Work out the finished part from the listing and answer in its coordinate system (mm). A direction names the side the tool comes from. Round coordinates to 2 decimals unless told otherwise and drop trailing zeros. Order: outer loops, then holes, each group sorted by start corner. A loop starts at its lowest first (then second) coordinate and runs counter-clockwise, first axis right, second up. Notation, with made-up numbers: (-14, 1) - (35, 1) arc R28 cw to (35, 25) - close; hole circle Ø9 at (-8.5, 27). An arc over 180 degrees is marked (long way). Answer in a Markdown table with one row per item.
from build123d import *

# Parameters (mm, degrees)
F1_W     = 279.4
F1_H     = 482.6
F1_W_2   = 221.90693
F1_H_2   = 17.004371
F1_H_3   = 15.303909
F1_H_4   = 15.30391
F2_DEPTH = 25.4


with BuildPart() as f2:
    # F1 (on face) → F2 (new body)
    with BuildSketch(Plane.XZ):
        Rectangle(F1_W, F1_H)
        with Locations((0, 130.508482)):
            Rectangle(F1_W_2, F1_H_2, mode=Mode.SUBTRACT)
        with Locations((0, 167.06787)):
            Rectangle(F1_W_2, F1_H_3, mode=Mode.SUBTRACT)
        with Locations((0, 202.777028)):
            Rectangle(F1_W_2, F1_H_4, mode=Mode.SUBTRACT)
    extrude(amount=F2_DEPTH)


solid = f2.part
1) The mould has two halves that part along X. Classify faces 1 (the face through (-2, -25.4, 3)), 2 (the face through (-2, -13, 122.006)), 3 (the face through (139.7, -13, -3)), 4 (the face through (-2, -13, 159.416)): released by +X, released by -X, zero draft, split by the parting line, or undercut.
Filled in:
| item | result |
|---|---|
| face 1 | zero draft |
| face 2 | undercut |
| face 3 | released by +X |
| face 4 | undercut |
2) Find section A-A, the plane x = 54. Give the vertices of the cut face in (y, z), then the cut area to 3 significant figures.
Filled in:
| item | result |
|---|---|
| outline | (-25.4, -241.3) - (0, -241.3) - (0, 122.01) - (-25.4, 122.01) - close; (-25.4, 139.01) - (0, 139.01) - (0, 159.42) - (-25.4, 159.42) - close; (-25.4, 174.72) - (0, 174.72) - (0, 195.13) - (-25.4, 195.13) - close; (-25.4, 210.43) - (0, 210.43) - (0, 241.3) - (-25.4, 241.3) - close |
| area | 11,000 mm^2 |
3) Which of the six approach directions +Z, -Z, +X, -X, +Y, -Y give full straight-line access (tool end or side, diameter ignored) to faces 5 (the face through (-110.953, -13, 130)), 6 (the face through (-2, -13, -241.3))?
Filled in:
| item | result |
|---|---|
| face 5 | +Y, -Y |
| face 6 | -Z, +X, -X, +Y, -Y |
4) Find the intervals of material crossed by probe 1 along Z at (x, y) = (-16, -9.5); probe 2 along X at (y, z) = (-19, 161.5), in increasing order. Write a range as from..to.
Filled in:
| item | result |
|---|---|
| probe 1 | z = -241.3..122.01, 139.01..159.42, 174.72..195.13, 210.43..241.3 |
| probe 2 | x = -139.7..-110.95, 110.95..139.7 |
5) Find section B-B, the plane y = -8. Give the vertices of the cut face in (x, z).
Filled in:
| item | result |
|---|---|
| outline | (-139.7, -241.3) - (139.7, -241.3) - (139.7, 241.3) - (-139.7, 241.3) - close; hole (-110.95, 122.01) - (110.95, 122.01) - (110.95, 139.01) - (-110.95, 139.01) - close; hole (-110.95, 159.42) - (110.95, 159.42) - (110.95, 174.72) - (-110.95, 174.72) - close; hole (-110.95, 195.13) - (110.95, 195.13) - (110.95, 210.43) - (-110.95, 210.43) - close |
6) This flat-tipped pin is pushed along its axis until it touches: pin 1 (6 mm diameter, centred on x = 88, z = 139.5, fed in from +Y). Where does it stop, or does it pass through?
Filled in:
| item | result |
|---|---|
| pin 1 | stops at y = 0 |
